from build123d import *

# Parameters (mm, degrees)
CHAMFER4_SIZE      = 4
CUT_EXTRUDE1_REACH = 92.2
SKETCH3_R          = 4


with BuildPart() as part:
    # Sketch2 → Revolve2 (revolve)
    with BuildSketch(Plane.XY, mode=Mode.PRIVATE) as revolve2_sk:
        with BuildLine():
            Line((-24, 0), (-24, 72))
            Line((-24, 72), (-36, 72))
            Line((-36, 72), (-36, 54))
            Line((-36, 54), (-34.882306768, 54))
            ThreePointArc((-34.882306768, 54), (-33.621047496, 53.601142721), (-32.558846616, 52.812732058))
            ThreePointArc((-32.558846616, 52.812732058), (-32.144965395, 52.173542011), (-32, 51.425981568))
            Line((-32, 51.425981568), (-32, 48))
            Line((-32, 48), (-54, 48))
            Line((-54, 48), (-54, 32))
            Line((-54, 32), (-32, 32))
            Line((-32, 32), (-32, 28))
            ThreePointArc((-32, 28), (-33.171572875, 25.171572875), (-36, 24))
            Line((-36, 24), (-36, 0))
            Line((-36, 0), (-24, 0))
        make_face()
    revolve(revolve2_sk.sketch.rotate(Axis((0, 0, 0), (0, 1, 0)), 270), axis=Axis((0, 0, 0), (0, 1, 0)))

    # Chamfer4
    chamfer4_edges = [part.edges().sort_by_distance(p)[0] for p in [
        (0, 0, 36),
        (0, 72, 36),
    ]]
    chamfer(chamfer4_edges, length=CHAMFER4_SIZE)

    # Sketch3 → Cut-Extrude1 (cut, up to next)
    with BuildSketch(Plane(origin=(0, 48, 0), x_dir=(1, 0, 0), z_dir=(0, 1, 0)), mode=Mode.PRIVATE) as cut_extrude1_sk1:
        with Locations(Location((44, 0, 0), (0, 0, 270))):
            Circle(SKETCH3_R)
    cut_extrude1_tool1 = extrude(cut_extrude1_sk1.sketch, amount=-CUT_EXTRUDE1_REACH, mode=Mode.PRIVATE) & part.part
    # Sketch3 → Cut-Extrude1 (cut, up to next)
    with BuildSketch(Plane(origin=(0, 48, 0), x_dir=(1, 0, 0), z_dir=(0, 1, 0)), mode=Mode.PRIVATE) as cut_extrude1_sk2:
        with Locations(Location((22, -38.105117767, 0), (0, 0, 270))):
            Circle(SKETCH3_R)
    cut_extrude1_tool2 = extrude(cut_extrude1_sk2.sketch, amount=-CUT_EXTRUDE1_REACH, mode=Mode.PRIVATE) & part.part
    # Sketch3 → Cut-Extrude1 (cut, up to next)
    with BuildSketch(Plane(origin=(0, 48, 0), x_dir=(1, 0, 0), z_dir=(0, 1, 0)), mode=Mode.PRIVATE) as cut_extrude1_sk3:
        with Locations(Location((-22, -38.105117767, 0), (0, 0, 270))):
            Circle(SKETCH3_R)
    cut_extrude1_tool3 = extrude(cut_extrude1_sk3.sketch, amount=-CUT_EXTRUDE1_REACH, mode=Mode.PRIVATE) & part.part
    # Sketch3 → Cut-Extrude1 (cut, up to next)
    with BuildSketch(Plane(origin=(0, 48, 0), x_dir=(1, 0, 0), z_dir=(0, 1, 0)), mode=Mode.PRIVATE) as cut_extrude1_sk4:
        with Locations(Location((-44, 0, 0), (0, 0, 270))):
            Circle(SKETCH3_R)
    cut_extrude1_tool4 = extrude(cut_extrude1_sk4.sketch, amount=-CUT_EXTRUDE1_REACH, mode=Mode.PRIVATE) & part.part
    # Sketch3 → Cut-Extrude1 (cut, up to next)
    with BuildSketch(Plane(origin=(0, 48, 0), x_dir=(1, 0, 0), z_dir=(0, 1, 0)), mode=Mode.PRIVATE) as cut_extrude1_sk5:
        with Locations(Location((-22, 38.105117767, 0), (0, 0, 270))):
            Circle(SKETCH3_R)
    cut_extrude1_tool5 = extrude(cut_extrude1_sk5.sketch, amount=-CUT_EXTRUDE1_REACH, mode=Mode.PRIVATE) & part.part
    # Sketch3 → Cut-Extrude1 (cut, up to next)
    with BuildSketch(Plane(origin=(0, 48, 0), x_dir=(1, 0, 0), z_dir=(0, 1, 0)), mode=Mode.PRIVATE) as cut_extrude1_sk6:
        with Locations(Location((22, 38.105117767, 0), (0, 0, 270))):
            Circle(SKETCH3_R)
    cut_extrude1_tool6 = extrude(cut_extrude1_sk6.sketch, amount=-CUT_EXTRUDE1_REACH, mode=Mode.PRIVATE) & part.part
    add(cut_extrude1_tool1.solids().sort_by_distance((44, 48, 0))[0], mode=Mode.SUBTRACT)
    add(cut_extrude1_tool2.solids().sort_by_distance((22, 48, 38.105118))[0], mode=Mode.SUBTRACT)
    add(cut_extrude1_tool3.solids().sort_by_distance((-22, 48, 38.105118))[0], mode=Mode.SUBTRACT)
    add(cut_extrude1_tool4.solids().sort_by_distance((-44, 48, 0))[0], mode=Mode.SUBTRACT)
    add(cut_extrude1_tool5.solids().sort_by_distance((-22, 48, -38.105118))[0], mode=Mode.SUBTRACT)
    add(cut_extrude1_tool6.solids().sort_by_distance((22, 48, -38.105118))[0], mode=Mode.SUBTRACT)


solid = part.part
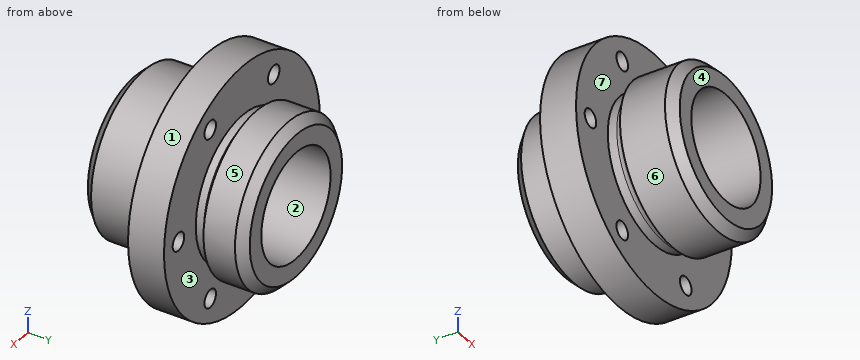
Source: CAD feature listing. Evaluate the final solid. Frame: model axes, mm. Face numbers are marked on the shaded views. A direction names the side the tool comes from. Round coordinates to 2 decimals unless told otherwise and drop trailing zeros. Write each loop counter-clockwise with the first axis right and the second up, starting at its lowest first coordinate (ties: lowest second). Pieces come first, ordered by that corner, then holes. Notation, with made-up numbers: M 64.5,43 L 103.5,43 A17 ccw 103.5,64 Z; hole C 2.5,-40 d7. An arc over 180 degrees is marked long. One line per item, written item: value. Start each with the question number.
Item 1: Ray query, L1, parallel to Z at x = 1, y = 57; L2, parallel to Y at x = -28, z = 21.5. Return the intervals inside material, ascending. Write a range as from..to.
Item 2: Section query C-C (z = 0). State how many separate pieces and enclosed holes the cut face has, plus the area to 3 significant figures.
Item 3: Section query B-B (x = -44). Return the cut outline in (y, z).
Item 4: Pin query (flat end, axial travel): pin 1 (1 mm diameter, centred on x = 18.5, y = 19, fed in from -Z); pin 2 (9 mm diameter, centred on x = 44, z = 0, fed in from -Y); pin 3 (4 mm diameter, centred on x = 13.5, z = -35, fed in from +Y). Return the tip coordinate at first contact, or that it passes through.
Item 5: Mould query, pull axis Z, two halves, no side actions, for the marked faces 1, 2 and 3. Classes: pulls with the +Z half, pulls with the -Z half, needs draft (parallel to the pull), parting line crosses it, or undercut.
Item 6: Set-up query: the marked faces 4, 5, 6 and 7. Return all of +Z, -Z, +X, -X, +Y, -Y with unobstructed straight access to the full face (end or side cutting, diameter ignored); none if empty.
Item 7: Section query A-A (y = 39). Return the cut outline in (x, z), plus the area to 3 significant figures.
Item 8: Section query D-D (y = 11). Return the cut outline in (x, z).
Result set:
1. L1: z = -35.99..-23.98, 23.98..35.99
1. L2: y = 3.3..24.06, 32..48, 54..68.7
2. separate pieces: 4
2. enclosed holes: 0
2. area: 1,910 mm²
3. outline: M 32,-31.3 L 48,-31.3 L 48,-4 L 32,-4 Z; M 32,4 L 48,4 L 48,31.3 L 32,31.3 Z
4. pin 1: stops at z = -31.18
4. pin 2: stops at y = 32
4. pin 3: stops at y = 68.49
5. face 1: parting line crosses it
5. face 2: undercut
5. face 3: needs draft
6. face 4: +Z, -Z, +X, -X, -Y
6. face 5: +Y
6. face 6: -Y
6. face 7: none
7. outline: C 0,0 d108; hole C -44,0 d8; hole C -22,-38.11 d8; hole C -22,38.11 d8; hole C 0,0 d48; hole C 22,-38.11 d8; hole C 22,38.11 d8; hole C 44,0 d8
7. area: 7,050 mm²
8. outline: C 0,0 d72; hole C 0,0 d48
